For this review, take the finished solid that the model builds, in its own axes (mm). Face numbers are marked on the shaded views. Give positions to 0.01 mm unless a question says otherwise; leave off trailing zeros. Write each loop counter-clockwise with the first axis right and the second up, starting at its lowest first coordinate (ties: lowest second). Pieces come first, ordered by that corner, then holes. Notation, with made-up numbers: (-22.75, 55.5) -> (33.25, 55.5) arc R12 cw to (33.25, 67.5) -> close; hole circle Ø5 at (2.5, 63.5). An arc over 180 degrees is marked (long way). Write item = value, one per line.
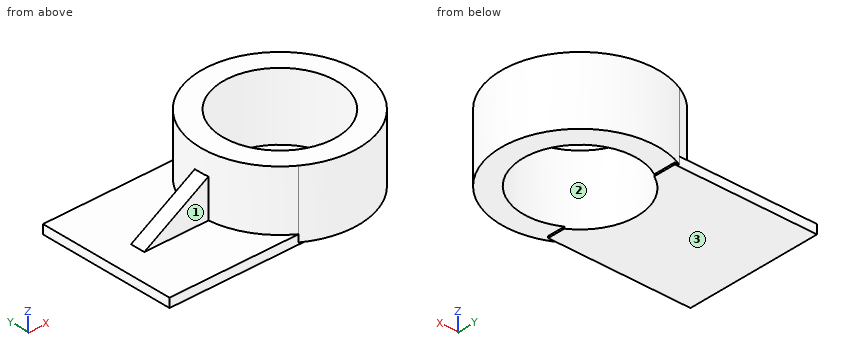
```python
from build123d import *

# Parameters (mm, degrees)
F0_W     = 56.8606331944
F0_H     = 37.3283550143
F0_H_2   = 39.9326570332
F0_W_2   = 23.0046827346
F1_DEPTH = 5.08
F2_R     = 44.2709641818
F3_DEPTH = 33.528
F4_DEPTH = 4.064
F5_DEPTH = 123.698
F7_DEPTH = 4.318
F8_DEPTH = 3.81


with BuildPart() as f1:
    # F0 (on Top) → F1 (new body)
    with BuildSketch(Plane.XY):
        with Locations((-28.4303165972, -18.6641775072)):
            Rectangle(F0_W, F0_H)
        with Locations((-28.4303165972, 19.9663285166)):
            Rectangle(F0_W, F0_H_2)
        with Locations((11.5023413673, 19.9663285166)):
            Rectangle(F0_W_2, F0_H_2)
        with Locations((11.5023413673, -18.6641775072)):
            Rectangle(F0_W_2, F0_H)
    extrude(amount=-F1_DEPTH)

    # F2 (on face) → F3 (join)
    with BuildSketch(Plane.XY):
        with Locations((39.4151285291, 0)):
            Circle(F2_R)
        with BuildLine():
            ThreePointArc((7.4318216845, 0), (39.4151285291, 31.9833068446), (71.3984353737, 0))
            ThreePointArc((71.3984353737, 0), (39.4151285291, -31.9833068446), (7.4318216845, 0))
        make_face(mode=Mode.SUBTRACT)
        with BuildLine():
            ThreePointArc((23.0046827346, -27.4523074721), (11.5961400498, -15.7808680594), (7.4318216845, 0))
            ThreePointArc((7.4318216845, 0), (11.5961400498, 15.7808680594), (23.0046827346, 27.4523074721))
            Line((23.0046827346, 27.4523074721), (23.0046827346, 39.9326570332))
            Line((23.0046827346, 39.9326570332), (20.3022749521, 39.9326570332))
            ThreePointArc((20.3022749521, 39.9326570332), (-4.7745397503, 2.6816947903), (15.6136121591, -37.3283550143))
            Line((15.6136121591, -37.3283550143), (23.0046827346, -37.3283550143))
            Line((23.0046827346, -37.3283550143), (23.0046827346, -27.4523074721))
        make_face()
    extrude(amount=F3_DEPTH)

    # F4 (add): a face of the model
    f4_faces = [f1.faces().sort_by_distance(p)[0] for p in [
        (60.1643011313, -37.8384648316, 0),
    ]]
    extrude(f4_faces, amount=F4_DEPTH)

    # F5 (cut): a face of the model
    f5_faces = [f1.faces().sort_by_distance(p)[0] for p in [
        (16.6239663947, 0, 0),
    ]]
    extrude(f5_faces, amount=-F5_DEPTH, mode=Mode.SUBTRACT)

    # F6 (on Front) → F7 (join)
    with BuildSketch(Plane.XZ):
        Polygon((-40.6748019159, 0), (0, 0), (0, 24.306833744), align=None)
    extrude(amount=F7_DEPTH)

    # F8 (add): a face of the model
    f8_faces = [f1.faces().sort_by_distance(p)[0] for p in [
        (-16.7954910738, 0, 7.1350124797),
    ]]
    extrude(f8_faces, amount=F8_DEPTH)


solid = f1.part
```
(1) The part is to be moulded in two halves that separate along Y. For the marked faces 1, 2 and 3, say which applies: released by +Y, released by -Y, zero draft, split by the parting line, or undercut.
Answers below:
face_1 = released by -Y
face_2 = undercut
face_3 = zero draft
(2) Take a section at D-D (z = 14.5). Write out the cut boundary in (x, y), plus the area to 3 significant figures.
Answers below:
outline = (-16.41, -4.32) -> (-4.64, -4.32) arc R44.27 ccw (long way) to (-4.86, 0) -> (-4.86, 3.81) -> (-16.41, 3.81) -> close; hole circle Ø63.97 at (39.42, 0)
area = 3,040 mm^2
(3) For pin 1 (4 mm diameter, centred on y = -2, z = 29, fed in from +X); pin 2 (1 mm diameter, centred on x = 0, z = 26.5, fed in from +Y); pin 3 (4 mm diameter, centred on x = -4.5, z = -3, fed in from -Y), all flat-tipped, find the tip position at first contact; note any pin that passes through.
Answers below:
pin_1 = 83.69
pin_2 = 21.11
pin_3 = -37.33
(4) To check wall thickness, follow probe 1 along X at (y, z) = (0, 24); probe 2 along Z at (x, y) = (-30.5, -24.5); probe 3 along Y at (x, z) = (-29, 1.5). State the ranges of each line that lie inside material, in increasing order.
Answers below:
probe_1 = -4.86 to 7.43, 71.4 to 83.69
probe_2 = -5.08 to 0
probe_3 = -4.32 to 3.81
(5) Take a section at C-C (z = -2). Write out the cut boundary in (x, y), plus the area to 3 significant figures.
Answers below:
outline = (-56.86, -37.33) -> (15.61, -37.33) arc R44.27 ccw (long way) to (20.3, 39.93) -> (-56.86, 39.93) -> close; hole circle Ø63.97 at (39.42, 0)
area = 7,470 mm^2
(6) Take a section at A-A (x = 45). Write out the cut boundary in (y, z), plus the area to 3 significant figures.
Answers below:
outline = (-43.92, -4.06) -> (-31.49, -4.06) -> (-31.49, 33.53) -> (-43.92, 33.53) -> close; (31.49, -4.06) -> (43.92, -4.06) -> (43.92, 33.53) -> (31.49, 33.53) -> close
area = 934 mm^2
(7) Take a section at B-B (y = 25.5). Write out the cut boundary in (x, z), plus the area to 3 significant figures.
Answers below:
outline = (-56.86, -5.08) -> (20.11, -5.08) -> (20.11, 33.53) -> (3.23, 33.53) -> (3.23, 0) -> (-56.86, 0) -> close; (58.72, -4.06) -> (75.6, -4.06) -> (75.6, 33.53) -> (58.72, 33.53) -> close
area = 1,590 mm^2
